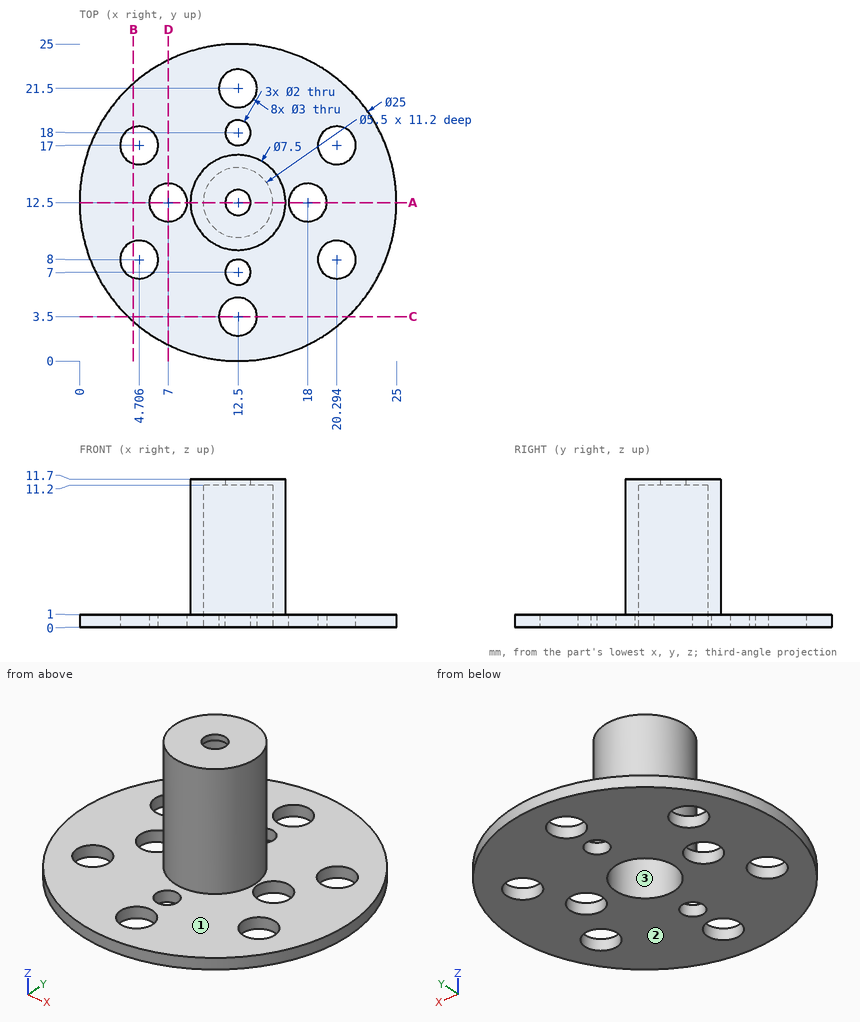
Design review of the part shown in the three views and the two pictorial views. Dimensions are in mm from the part's minimum x, y and z. A direction names the side the tool comes from. Coordinates: 2 decimals unless noted, no trailing zeros. Order: outer loops, then holes, each group sorted by start corner. A loop starts at its lowest first (then second) coordinate and runs counter-clockwise, first axis right, second up.
Item 1: For line 1 (Y direction, x = 12.5, z = 0.4); line 2 (X direction, y = 7, z = 0.6) (1 decimal); line 3 (Z direction, x = 9.5, y = 7.5), list the stretches that pass through material, from the lowest coordinate up.
Item 2: Take a section at A-A, the plane y = 12.5. Write out the cut boundary in (x, z).
Item 3: Take a section at C-C, the plane y = 3.5. Write out the cut boundary in (x, z) (1 decimal).
Item 4: For the marked faces 1, 2 and 3, list the 3-axis set-ups (+Z, -Z, +X, -X, +Y, -Y) from which the entire face can be reached by the end or side of a thin tool; tool diameter is ignored.
Item 5: For pin 1 Ø3 at (x, y) = (18.5, 19) entering from +Z; pin 2 Ø3 at (x, y) = (11.5, 13) entering from -Z; pin 3 Ø5 at (y, z) = (15, 2) entering from +X, all flat-tipped, find the tip position at first contact; note any pin that passes through.
Item 6: Take a section at D-D, the plane x = 7. Write out the cut boundary in (y, z) (3 decimals).
Item 7: Take a section at B-B, the plane x = 4.25. Write out the cut boundary in (y, z), then the cut area to 3 significant figures.
The answers:
1. line 1: y = 0 to 2, 5 to 6, 8 to 9.75, 15.25 to 17, 19 to 20, 23 to 25
1. line 2: x = 1.3 to 3.6, 5.8 to 11.5, 13.5 to 19.2, 21.4 to 23.7
1. line 3: z = 0 to 1
2. outline: (0, 0) - (5.5, 0) - (5.5, 1) - (0, 1) - close; (8.5, 0) - (9.75, 0) - (9.75, 11.2) - (11.5, 11.2) - (11.5, 11.7) - (8.75, 11.7) - (8.75, 1) - (8.5, 1) - close; (13.5, 11.2) - (15.25, 11.2) - (15.25, 0) - (16.5, 0) - (16.5, 1) - (16.25, 1) - (16.25, 11.7) - (13.5, 11.7) - close; (19.5, 0) - (25, 0) - (25, 1) - (19.5, 1) - close
3. outline: (3.8, 0) - (11, 0) - (11, 1) - (3.8, 1) - close; (14, 0) - (21.2, 0) - (21.2, 1) - (14, 1) - close
4. face 1: +Z
4. face 2: -Z, +X, -X, +Y, -Y
4. face 3: -Z
5. pin 1: stops at z = 1
5. pin 2: stops at z = 11.2
5. pin 3: stops at x = 25
6. outline: (1.275, 0) - (11, 0) - (11, 1) - (1.275, 1) - close; (14, 0) - (23.725, 0) - (23.725, 1) - (14, 1) - close
7. outline: (3.11, 0) - (6.57, 0) - (6.57, 1) - (3.11, 1) - close; (9.43, 0) - (15.57, 0) - (15.57, 1) - (9.43, 1) - close; (18.43, 0) - (21.89, 0) - (21.89, 1) - (18.43, 1) - close
7. area: 13.1 mm2
